Build history of the part. All positions in model axes, mm. Face numbers are marked on the shaded views. A direction names the side the tool comes from. Round coordinates to 2 decimals unless told otherwise and drop trailing zeros. Write each loop counter-clockwise with the first axis right and the second up, starting at its lowest first coordinate (ties: lowest second). Pieces come first, ordered by that corner, then holes. Notation, with made-up numbers: M -22,62 L 18,62 A7 cw 18,69 Z; hole C 81,-2 d2. An arc over 180 degrees is marked long. Write item = value, one per line.
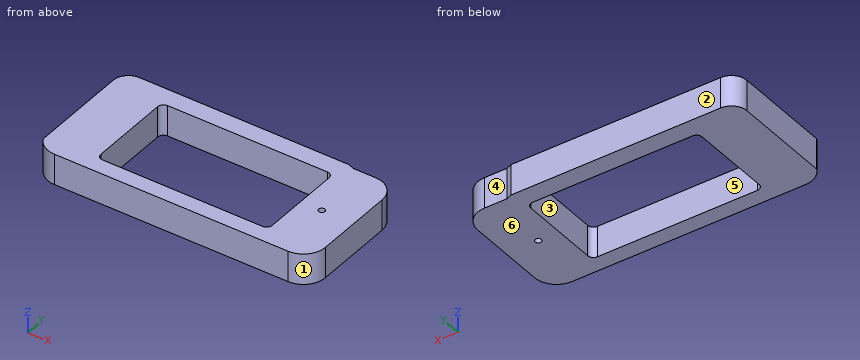
Autodesk Inventor part; units mm, degrees
ref_plane "YZ Plane" through (0, 0, 0) normal (1, 0, 0) x (0, 1, 0)
ref_plane "XZ Plane" through (0, 0, 0) normal (0, 1, 0) x (-1, 0, 0)
ref_plane "XY Plane" through (0, 0, 0) normal (0, 0, 1) x (1, 0, 0)
ref_plane "Płaszczyzna konstrukcyjna1" through (0, 0, 0) normal (0, 0, 1) x (1, 0, 0)
sketch "Szkic1" plane through (0, 0, 0) normal (0, 0, 1) x (1, 0, 0)
  line L0 (23.2, 1) -> (23.2, -9.5)
  arc A0 (23.2, 1) -> (20.35, 3.85) centre (20.35, 1) ccw
  line L1 (20.35, 3.85) -> (17.375, 3.85)
  line L2 (17.375, 3.85) -> (16.7, 4.15)
  line L3 (16.7, 4.15) -> (-6.1, 4.15)
  line L4 (-6.1, 4.15) -> (-6.1, 2.15)
  line L5 (16.7, 2.15) -> (-6.1, 2.15)
  line L6 (16.7, -10.75) -> (16.7, 2.15)
  line L7 (16.7, -10.75) -> (-12.6112, -10.75)
  arc A1 (-12.6112, -10.75) -> (-10.05, -12.35) centre (-10.05, -9.5) ccw
  line L8 (-10.05, -12.35) -> (20.35, -12.35)
  arc A2 (20.35, -12.35) -> (23.2, -9.5) centre (20.35, -9.5) ccw
  circle A3 centre (19.05, -4.25) radius 0.4
  line L9 (-5.25, 1.85) -> (-10.05, 1.85)
  line L10 (-10.9, 1) -> (-10.9, -3.7)
  arc A4 (-10.05, 1.85) -> (-10.9, 1) centre (-10.05, 1) ccw
  line L11 (-10.9, -4.8) -> (-10.9, -9.5)
  arc A5 (-10.9, -9.5) -> (-10.05, -10.35) centre (-10.05, -9.5) ccw
  line L12 (-10.05, -10.35) -> (-5.25, -10.35)
  line L13 (-12.6112, -10.75) -> (-12.6112, 2.15)
  line L14 (-10.6112, 4.15) -> (-6.1, 4.15)
  arc A6 (-10.6112, 4.15) -> (-12.6112, 2.15) centre (-10.6112, 2.15) ccw
  line L15 (-2.55, 1.95) -> (12.85, 1.95)
  line L16 (12.85, -10.45) -> (-2.55, -10.45)
  line L17 (-2.55, -10.45) -> (-10.05, -10.35)
  line L18 (12.85, -10.45) -> (16.7, -10.45)
  line L19 (12.85, 1.95) -> (16.7, 1.95)
  line L20 (-2.55, 1.95) -> (-5.25, 1.85)
  line L21 (-10.9, -3.7) -> (-10.9, -4.8)
  line L22 (16.3, 1) -> (16.3, -9.5)
  arc A7 (15.55, -10.25) -> (16.3, -9.5) centre (15.55, -9.5) ccw
  line L23 (15.55, -10.25) -> (-5.25, -10.25)
  arc A8 (-6, -9.5) -> (-5.25, -10.25) centre (-5.25, -9.5) ccw
  line L24 (-6, -9.5) -> (-6, 1)
  arc A9 (-5.25, 1.75) -> (-6, 1) centre (-5.25, 1) ccw
  line L25 (-5.25, 1.75) -> (15.55, 1.75)
  arc A10 (16.3, 1) -> (15.55, 1.75) centre (15.55, 1) ccw
  line L26 (-1.9, -0.65) -> (1.2, -0.65)
  line L27 (-1.9, -1.75) -> (-1.9, -0.65)
  line L28 (1.2, -1.75) -> (-1.9, -1.75)
  line L29 (1.2, -0.65) -> (1.2, -1.75)
  line L30 (5.4, 0.75) -> (5.4, 0.4385)
  arc A11 (5.4, 0.75) -> (5.4, -2.85) centre (5.8571, -1.05) ccw
  line L31 (5.4, -2.5385) -> (5.4, -2.85)
  arc A12 (4.3078, -1.2057) -> (5.4, -2.5385) centre (5.8571, -1.05) ccw
  line L32 (5.4, -1.2057) -> (4.3078, -1.2057)
  line L33 (5.4, -0.8943) -> (5.4, -1.2057)
  line L34 (4.3078, -0.8943) -> (5.4, -0.8943)
  arc A13 (5.4, 0.4385) -> (4.3078, -0.8943) centre (5.8571, -1.05) ccw
  line L35 (3.9, 0.75) -> (3.9, 0.4385)
  arc A14 (3.9, 0.75) -> (3.9, -2.85) centre (4.3571, -1.05) ccw
  line L36 (3.9, -2.5385) -> (3.9, -2.85)
  arc A15 (3.9, 0.4385) -> (3.9, -2.5385) centre (4.3571, -1.05) ccw
  circle A16 centre (-4.75, -8.6) radius 1
  circle A17 centre (15.05, -8.6) radius 1
  circle A18 centre (15.05, 0.1) radius 1
  circle A19 centre (-4.75, 0.1) radius 1
  line L37 (10.7377, -7.5396) -> (10.2468, -7.5396)
  line L38 (10.2468, -7.5396) -> (10.2468, -7.75)
  line L39 (10.2468, -7.75) -> (11.4156, -7.75)
  line L40 (11.4156, -7.75) -> (11.4156, -7.5396)
  line L41 (11.4156, -7.5396) -> (10.9247, -7.5396)
  line L42 (10.9247, -7.5396) -> (10.9247, -5.95)
  line L43 (10.9247, -5.95) -> (10.7377, -5.95)
  line L44 (10.7377, -5.95) -> (10.7377, -7.5396)
  line L45 (11.626, -7.75) -> (12.1804, -7.75)
  spline S0 degree 3 poles (12.1804, -7.75) (12.1963, -7.75) (12.2267, -7.75) (12.2708, -7.7479) (12.3118, -7.7457) (12.3495, -7.7415) (12.384, -7.7369) (12.4153, -7.7312) (12.4433, -7.7239) (12.4607, -7.7181) (12.469, -7.7153) knots 0 0 0 0 0.162643 0.312901 0.453294 0.58413 0.70285 0.811058 0.910586 1 1 1 1
  spline S1 degree 3 poles (12.469, -7.7153) (12.4794, -7.7113) (12.5003, -7.7032) (12.5297, -7.6872) (12.5577, -7.6693) (12.5841, -7.6488) (12.6087, -7.6256) (12.6318, -7.6) (12.653, -7.5717) (12.6725, -7.5411) (12.6907, -7.5086) (12.7057, -7.4738) (12.7192, -7.4375) (12.7294, -7.3991) (12.7381, -7.3591) (12.7436, -7.3172) (12.7476, -7.2734) (12.7479, -7.2436) (12.7481, -7.2284) knots 0 0 0 0 0.056072 0.112012 0.167171 0.222811 0.27891 0.336355 0.395158 0.456072 0.518045 0.581404 0.645662 0.712108 0.780061 0.850885 0.92373 1 1 1 1
  spline S2 degree 3 poles (12.7481, -7.2284) (12.7477, -7.2084) (12.7471, -7.1693) (12.7412, -7.1122) (12.7313, -7.058) (12.7179, -7.0065) (12.7004, -6.9578) (12.6787, -6.912) (12.6533, -6.8689) (12.6243, -6.8285) (12.5902, -6.7918) (12.5498, -6.7603) (12.5042, -6.7334) (12.4527, -6.7121) (12.3959, -6.6948) (12.3332, -6.683) (12.2648, -6.6762) (12.2175, -6.6752) (12.1929, -6.6747) knots 0 0 0 0 0.066633 0.130318 0.191414 0.250222 0.307644 0.363778 0.418941 0.474177 0.529339 0.585724 0.64416 0.705484 0.771261 0.841987 0.917917 1 1 1 1
  line L46 (12.1929, -6.6747) -> (11.813, -6.6747)
  line L47 (11.813, -6.6747) -> (11.813, -5.95)
  line L48 (11.813, -5.95) -> (11.626, -5.95)
  line L49 (11.626, -5.95) -> (11.626, -7.75)
  line L50 (-2.2056, -2.52) -> (-2.1, -2.4134)
  line L51 (-0.9587, -3.7548) -> (-2.2056, -2.52)
  line L52 (-1.121, -5.7025) -> (-0.9587, -3.7548)
  line L53 (-2.2056, -6.7765) -> (-1.121, -5.7025)
  line L54 (-2.1, -6.8831) -> (-2.2056, -6.7765)
  line L55 (-1.1402, -5.9326) -> (-2.1, -6.8831)
  line L56 (-1.1875, -6.5) -> (-1.1402, -5.9326)
  line L57 (-1.1875, -6.5) -> (-1.5, -6.5)
  line L58 (-1.5, -6.65) -> (-1.5, -6.5)
  line L59 (-1.2, -6.65) -> (-1.5, -6.65)
  arc A20 (-1.2, -6.65) -> (1.2, -6.65) centre (0, -5.75) ccw
  line L60 (1.2, -6.65) -> (1.2, -6.15)
  line L61 (1.2, -6.15) -> (1.4598, -6.15)
  line L62 (2.2, -6.8831) -> (1.4598, -6.15)
  line L63 (2.3056, -6.7765) -> (2.2, -6.8831)
  line L64 (1.6, -6.0778) -> (2.3056, -6.7765)
  line L65 (1.6, -6.0778) -> (1.6, -5.45)
  line L66 (1.2, -5.45) -> (1.6, -5.45)
  line L67 (1.2, -5.45) -> (1.2, -3.6149)
  line L68 (2.3056, -2.52) -> (1.2, -3.6149)
  line L69 (2.2, -2.4134) -> (2.3056, -2.52)
  line L70 (1.3978, -3.2079) -> (2.2, -2.4134)
  arc A21 (1.3978, -3.2079) -> (0.6536, -3.05) centre (1, -3.25) ccw
  line L71 (0.6536, -3.05) -> (-0.75, -3.05)
  line L72 (-0.75, -3.05) -> (-0.75, -2.75)
  line L73 (-0.9, -2.75) -> (-0.75, -2.75)
  line L74 (-0.9, -3.05) -> (-0.9, -2.75)
  line L75 (-0.9425, -3.5598) -> (-0.9, -3.05)
  line L76 (-2.1, -2.4134) -> (-0.9425, -3.5598)
  point P0 (0, 0)
  point P1 (-12.6112, 4.15)
  dimension "d0" = 2
extrude "Wyciągnięcie proste1" add sketch "Szkic1" along normal blind 4 contours L0 A2 L8 A1 L7 L6 L5 L4 L3 L2 L1 A0 | L13 A6 L14 L4 L5 L6 L19 L15 L20 L9 A4 L10 L21 L11 A5 L17 L16 L18 L7 | L18 L16 L17 A5 L11 L21 L10 A4 L9 L20 L15 L19 L6
properties part number "ServoPlate"
1. Band-saw the part on A-A (x = 19.05). List the corners of the cut face in (y, z), plus the area to 3 significant figures.
Responses:
outline = M -12.35,0 L -4.65,0 L -4.65,4 L -12.35,4 Z; M -3.85,0 L 3.85,0 L 3.85,4 L -3.85,4 Z
area = 61.6 mm²
2. Flat gauge pins, fed straight in: pin 1 (1.5 mm diameter, centred on x = -4, y = -8, fed in from -Z); pin 2 (0.9 mm diameter, centred on x = 19, z = 2, fed in from +Y). Where does each tip first touch, or does it go through?
Responses:
pin_1 = through
pin_2 = 3.85
3. Tool access for the marked faces 4, 5 and 6: list every direction of +Z, -Z, +X, -X, +Y, -Y with a clear straight run to the whole face (end or side of a thin tool).
Responses:
face_4 = +Z, -Z, +X, +Y
face_5 = +Z, -Z
face_6 = -Z, +X, -X, +Y, -Y
4. Band-saw the part on C-C (z = 1.35). List the corners of the cut face in (x, y) (3 decimals).
Responses:
outline = M -12.611,-10.75 A2.85 ccw -10.05,-12.35 L 20.35,-12.35 A2.85 ccw 23.2,-9.5 L 23.2,1 A2.85 ccw 20.35,3.85 L 17.375,3.85 L 16.7,4.15 L -10.611,4.15 A2 ccw -12.611,2.15 Z; hole M -6,-9.5 A0.75 ccw -5.25,-10.25 L 15.55,-10.25 A0.75 ccw 16.3,-9.5 L 16.3,1 A0.75 ccw 15.55,1.75 L -5.25,1.75 A0.75 ccw -6,1 Z; hole C 19.05,-4.25 d0.8
5. Mould opens along Y. For the marked faces 1, 2 and 3 say: pulls with the +Y half, pulls with the -Y half, needs draft (parallel to the pull), parting line crosses it, or undercut.
Responses:
face_1 = pulls with the -Y half
face_2 = pulls with the +Y half
face_3 = undercut
6. Band-saw the part on B-B (y = -5.75). List the corners of the cut face in (x, z), plus the area to 3 significant figures.
Responses:
outline = M -12.61,0 L -6,0 L -6,4 L -12.61,4 Z; M 16.3,0 L 23.2,0 L 23.2,4 L 16.3,4 Z
area = 54.0 mm²
7. Probe probe 1 along Y at (x, z) = (19.05, 2.5); probe 2 along X at (y, z) = (1, 2.1); probe 3 along Y at (x, z) = (12.5, 1.65). List the from-to ranges inside material, lowest first.
Responses:
probe_1 = -12.35 to -4.65, -3.85 to 3.85
probe_2 = -12.61 to -6, 16.3 to 23.2
probe_3 = -12.35 to -10.25, 1.75 to 4.15
